For this review, take the finished solid that the model builds, in its own axes (mm). Round coordinates to 2 decimals unless told otherwise and drop trailing zeros. Order: outer loops, then holes, each group sorted by start corner. A loop starts at its lowest first (then second) coordinate and runs counter-clockwise, first axis right, second up. Notation, with made-up numbers: M 39,50.25 L 61,50.25 A15 cw 61,77.25 Z; hole C -18,-39.5 d11. An arc over 180 degrees is marked long. Use a Markdown table: item, result.
from build123d import *

# Parameters (mm, degrees)
SKETCH1_W           = 55
SKETCH1_H           = 16
SKETCH1_R           = 2
BOSS_EXTRUDE1_DEPTH = 5
SKETCH2_W           = 55
SKETCH2_H           = 3
BOSS_EXTRUDE2_DEPTH = 3
SKETCH4_W           = 55
SKETCH4_H           = 16
SKETCH4_R           = 2
BOSS_EXTRUDE3_DEPTH = 5
SKETCH5_W           = 55
SKETCH5_H           = 3
BOSS_EXTRUDE4_DEPTH = 3
BOSS_EXTRUDE5_DEPTH = 5
SKETCH7_W           = 3
SKETCH7_H           = 75
BOSS_EXTRUDE6_DEPTH = 3
SKETCH8_R           = 2
CUT_EXTRUDE2_DEPTH  = 5
SKETCH10_R          = 4
CUT_EXTRUDE3_DEPTH  = 2
SKETCH11_R          = 2
CUT_EXTRUDE4_DEPTH  = 5
SKETCH12_R          = 2
CUT_EXTRUDE5_DEPTH  = 5
FILLET1_R           = 5


with BuildPart() as part:
    # Sketch1 → Boss-Extrude1 (new body)
    with BuildSketch(Plane(origin=(0, 0, 0), x_dir=(1, 0, 0), z_dir=(0, 1, 0))):
        with Locations((-8.751560295, 3.021428571)):
            Rectangle(SKETCH1_W, SKETCH1_H)
        with Locations(Location((-6.751560295, 3.021428571, 0), (0, 0, 270))):
            Circle(SKETCH1_R, mode=Mode.SUBTRACT)
        with Locations(Location((-19.251560295, 3.021428571, 0), (0, 0, 270))):
            Circle(SKETCH1_R, mode=Mode.SUBTRACT)
    extrude(amount=BOSS_EXTRUDE1_DEPTH)

    # Sketch2 → Boss-Extrude2 (add)
    with BuildSketch(Plane(origin=(0, 5, 0), x_dir=(1, 0, 0), z_dir=(0, 1, 0))):
        with Locations((-8.751560295, 9.521428571)):
            Rectangle(SKETCH2_W, SKETCH2_H)
        with Locations((-8.751560295, -3.478571429)):
            Rectangle(SKETCH2_W, SKETCH2_H)
    extrude(amount=BOSS_EXTRUDE2_DEPTH)



with BuildPart() as body_2:
    # Sketch4 → Boss-Extrude3 (new body)
    with BuildSketch(Plane.XZ):
        with Locations((-8.751560295, 87.978571429)):
            Rectangle(SKETCH4_W, SKETCH4_H)
        with Locations(Location((-19.251560295, 87.978571429, 0), (0, 0, 270))):
            Circle(SKETCH4_R, mode=Mode.SUBTRACT)
        with Locations(Location((-6.751560295, 87.978571429, 0), (0, 0, 270))):
            Circle(SKETCH4_R, mode=Mode.SUBTRACT)
    extrude(amount=-BOSS_EXTRUDE3_DEPTH)

    # Sketch5 → Boss-Extrude4 (add)
    with BuildSketch(Plane(origin=(0, 5, 0), x_dir=(1, 0, 0), z_dir=(0, 1, 0))):
        with Locations((-8.751560295, -94.478571429)):
            Rectangle(SKETCH5_W, SKETCH5_H)
        with Locations((-8.751560295, -81.478571429)):
            Rectangle(SKETCH5_W, SKETCH5_H)
    extrude(amount=BOSS_EXTRUDE4_DEPTH)


with BuildPart() as part_1:
    add(part.part)

    add(body_2.part)  # Boss-Extrude5 merges body 2
    # Sketch6 → Boss-Extrude5 (add)
    with BuildSketch(Plane.XZ):
        Polygon((-6.751560295, 79.978571429), (1.248439705, 79.978571429), (1.248439705, 4.978571429), (-14.751560295, 4.978571429), (-14.751560295, 79.978571429), align=None)
    extrude(amount=-BOSS_EXTRUDE5_DEPTH)

    # Sketch7 → Boss-Extrude6 (add)
    with BuildSketch(Plane(origin=(0, 5, 0), x_dir=(1, 0, 0), z_dir=(0, 1, 0))):
        with Locations((-0.251560295, -42.478571429)):
            Rectangle(SKETCH7_W, SKETCH7_H)
        with Locations((-13.251560295, -42.478571429)):
            Rectangle(SKETCH7_W, SKETCH7_H)
    extrude(amount=BOSS_EXTRUDE6_DEPTH)

    # Sketch8 → Cut-Extrude2 (cut)
    with BuildSketch(Plane.XZ):
        with Locations(Location((13.748439705, -3.021428571, 0), (0, 0, 270))):
            Circle(SKETCH8_R)
        with Locations(Location((13.748439705, 87.978571429, 0), (0, 0, 270))):
            Circle(SKETCH8_R)
    extrude(amount=-CUT_EXTRUDE2_DEPTH, mode=Mode.SUBTRACT)

    # Sketch10 → Cut-Extrude3 (cut)
    with BuildSketch(Plane.XZ):
        with Locations(Location((-19.251560295, -3.021428571, 0), (0, 0, 270))):
            Circle(SKETCH10_R)
        with Locations(Location((-6.751560295, -3.021428571, 0), (0, 0, 270))):
            Circle(SKETCH10_R)
        with Locations(Location((13.748439705, -3.021428571, 0), (0, 0, 270))):
            Circle(SKETCH10_R)
        with Locations(Location((-19.251560295, 87.978571429, 0), (0, 0, 270))):
            Circle(SKETCH10_R)
        with Locations(Location((-6.751560295, 87.978571429, 0), (0, 0, 270))):
            Circle(SKETCH10_R)
        with Locations(Location((13.748439705, 87.978571429, 0), (0, 0, 270))):
            Circle(SKETCH10_R)
    extrude(amount=-CUT_EXTRUDE3_DEPTH, mode=Mode.SUBTRACT)

    # Sketch11 → Cut-Extrude4 (cut)
    with BuildSketch(Plane.XZ):
        with Locations(Location((-31.251560295, -3.021428571, 0), (0, 0, 270))):
            Circle(SKETCH11_R)
        with Locations(Location((-31.251560295, 87.978571429, 0), (0, 0, 270))):
            Circle(SKETCH11_R)
    extrude(amount=-CUT_EXTRUDE4_DEPTH, mode=Mode.SUBTRACT)

    # Sketch12 → Cut-Extrude5 (cut)
    with BuildSketch(Plane(origin=(0, 5, 0), x_dir=(1, 0, 0), z_dir=(0, 1, 0))):
        with Locations(Location((-6.751560295, -12.478571429, 0), (0, 0, 270))):
            Circle(SKETCH12_R)
        with Locations(Location((-6.751560295, -22.478571429, 0), (0, 0, 270))):
            Circle(SKETCH12_R)
        with Locations(Location((-6.751560295, -32.478571429, 0), (0, 0, 270))):
            Circle(SKETCH12_R)
        with Locations(Location((-6.751560295, -42.478571429, 0), (0, 0, 270))):
            Circle(SKETCH12_R)
        with Locations(Location((-6.751560295, -52.478571429, 0), (0, 0, 270))):
            Circle(SKETCH12_R)
        with Locations(Location((-6.751560295, -62.478571429, 0), (0, 0, 270))):
            Circle(SKETCH12_R)
        with Locations(Location((-6.751560295, -72.478571429, 0), (0, 0, 270))):
            Circle(SKETCH12_R)
    extrude(amount=-CUT_EXTRUDE5_DEPTH, mode=Mode.SUBTRACT)

    # Fillet1
    fillet1_edges = [part_1.edges().sort_by_distance(p)[0] for p in [
        (-14.751560295, 4, 79.978571429),
        (1.248439705, 4, 79.978571429),
        (1.248439705, 4, 4.978571429),
        (-14.751560295, 4, 4.978571429),
    ]]
    fillet(fillet1_edges, radius=FILLET1_R)


solid = part_1.part
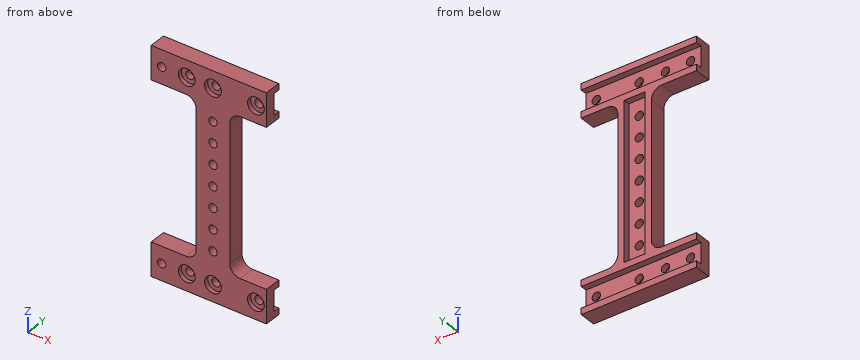
Q1. Add section D-D (z = 59.5). Write out the cut boundary in (x, y).
Determined:
| item | result |
|---|---|
| outline | M -14.75,0 L 1.25,0 L 1.25,8 L -1.75,8 L -1.75,5 L -11.75,5 L -11.75,8 L -14.75,8 Z |
Q2. Clearance check with flat-ended pins moving along their axes: pin 1 (6.5 mm diameter, centred on x = 13.5, z = -3.5, fed in from -Y); pin 2 (4.5 mm diameter, centred on x = -6.75, z = 52.48, fed in from +Y); pin 3 (9 mm diameter, centred on x = -6.5, z = -4.5, fed in from -Y); pin 4 (0.9 mm diameter, centred on y = 6.5, z = 46, fed in from +X). State where each tip first meets the part, or that it passes through.
Determined:
| item | result |
|---|---|
| pin 1 | stops at y = 2 |
| pin 2 | stops at y = 5 |
| pin 3 | stops at y = 0 |
| pin 4 | stops at x = 1.25 |
Q3. Wall thickness on line 1 along Z through (x, y) = (-8, 7.5); line 2 along X through (y, z) = (6.25, 21); line 3 along Z through (x, y) = (13.5, 1): over which ranges is each line inside the solid? List them lowest first. Write a range as [from, to].
Determined:
| item | result |
|---|---|
| line 1 | z = [-11.02, -8.02], [1.98, 4.98], [79.98, 82.98], [92.98, 95.98] |
| line 2 | x = [-14.75, -11.75], [-1.75, 1.25] |
| line 3 | z = [-11.02, -7.01], [0.97, 4.98], [79.98, 83.99], [91.97, 95.98] |
Q4. Add section B-B (x = -28). Write out the cut boundary in (y, z).
Determined:
| item | result |
|---|---|
| outline | M 0,-11.02 L 8,-11.02 L 8,-8.02 L 5,-8.02 L 5,1.98 L 8,1.98 L 8,4.98 L 0,4.98 Z; M 0,79.98 L 8,79.98 L 8,82.98 L 5,82.98 L 5,92.98 L 8,92.98 L 8,95.98 L 0,95.98 Z |
Q5. Add section A-A (y = 6.25). Write out the cut boundary in (x, z), then the cut area to 3 significant figures.
Determined:
| item | result |
|---|---|
| outline | M -36.25,-11.02 L 18.75,-11.02 L 18.75,-8.02 L -36.25,-8.02 Z; M -36.25,1.98 L 18.75,1.98 L 18.75,4.98 L 6.25,4.98 A5 cw 1.25,9.98 L 1.25,74.98 A5 cw 6.25,79.98 L 18.75,79.98 L 18.75,82.98 L -36.25,82.98 L -36.25,79.98 L -19.75,79.98 A5 cw -14.75,74.98 L -14.75,9.98 A5 cw -19.75,4.98 L -36.25,4.98 Z; M -36.25,92.98 L 18.75,92.98 L 18.75,95.98 L -36.25,95.98 Z; hole M -11.75,4.98 L -1.75,4.98 L -1.75,79.98 L -11.75,79.98 Z |
| area | 1,130 mm^2 |
Q6. Add section C-C (z = 22). Write out the cut boundary in (x, y).
Determined:
| item | result |
|---|---|
| outline | M -14.75,0 L -8.69,0 L -8.69,5 L -11.75,5 L -11.75,8 L -14.75,8 Z; M -4.81,0 L 1.25,0 L 1.25,8 L -1.75,8 L -1.75,5 L -4.81,5 Z |
